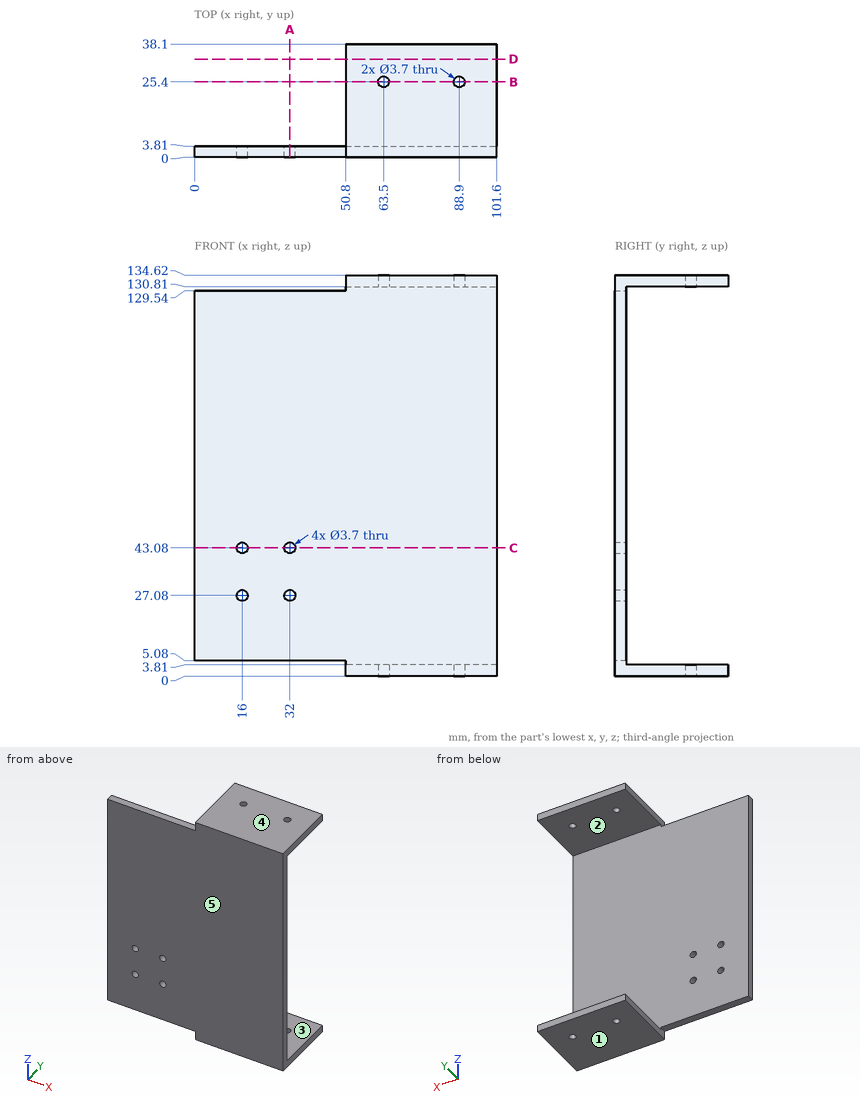
Part print with two shaded views. Sizes in mm from the minimum x, y, z corner. A direction names the side the tool comes from. Coordinates: 2 decimals unless noted, no trailing zeros. Order: outer loops, then holes, each group sorted by start corner. A loop starts at its lowest first (then second) coordinate and runs counter-clockwise, first axis right, second up. Notation, with made-up numbers: M 61.25,51 L 105.25,51 A33 ccw 105.25,87 Z; hole C -24.75,62.25 d9. An arc over 180 degrees is marked long. One line per question, with ' | ' between items. Start each with the question number.
1. Cut at D-D (y = 33). Write the cut outline in (x, z), plus the area to 3 significant figures.
2. Cut at B-B (y = 25.4). Write the cut outline in (x, z).
3. Mould opens along Z. For the marked faces 3, 4 and 5 say: +Z half, -Z half, draft (parallel to the pull), parting line (faces both ways), or undercut.
4. Tool access for the marked faces 1 and 2: list every direction of +Z, -Z, +X, -X, +Y, -Y with a clear straight run to the whole face (end or side of a thin tool).
5. Cut at A-A (x = 32). Write the cut outline in (y, z), plus the area to 3 significant figures.
6. Cut at C-C (z = 43.08). Write the cut outline in (x, y).
7. Flat gauge pins, fed straight in: P1, Ø2, axis at x = 88.9, y = 25.4, coming from the -Z side; P2, Ø2.5, axis at y = 27.5, z = 132, coming from the -X side; P3, Ø5, axis at x = 32, z = 27.08, coming from the +Y side; P4, Ø1.9, axis at x = 28.5, y = 1.5, coming from the -Z side. Where does each tip first touch, or does it go through?
8. Wall check: line 1 along X through (y, z) = (1.35, 43.08); line 2 along X through (y, z) = (25.4, 2.25); line 3 along Z through (x, y) = (16, 2.2). Give the ranges that are in metal, low to high. Write a range as [from, to].
The answers:
1) outline: M 50.8,0 L 101.6,0 L 101.6,3.81 L 50.8,3.81 Z; M 50.8,130.81 L 101.6,130.81 L 101.6,134.62 L 50.8,134.62 Z | area: 387 mm2
2) outline: M 50.8,0 L 61.65,0 L 61.65,3.81 L 50.8,3.81 Z; M 50.8,130.81 L 61.65,130.81 L 61.65,134.62 L 50.8,134.62 Z; M 65.35,0 L 87.05,0 L 87.05,3.81 L 65.35,3.81 Z; M 65.35,130.81 L 87.05,130.81 L 87.05,134.62 L 65.35,134.62 Z; M 90.75,0 L 101.6,0 L 101.6,3.81 L 90.75,3.81 Z; M 90.75,130.81 L 101.6,130.81 L 101.6,134.62 L 90.75,134.62 Z
3) face 3: undercut | face 4: +Z half | face 5: draft
4) face 1: -Z, +X, -X, +Y, -Y | face 2: +X, -X, +Y
5) outline: M 0,5.08 L 3.81,5.08 L 3.81,25.23 L 0,25.23 Z; M 0,28.93 L 3.81,28.93 L 3.81,41.23 L 0,41.23 Z; M 0,44.93 L 3.81,44.93 L 3.81,129.54 L 0,129.54 Z | area: 446 mm2
6) outline: M 0,0 L 14.15,0 L 14.15,3.81 L 0,3.81 Z; M 17.85,0 L 30.15,0 L 30.15,3.81 L 17.85,3.81 Z; M 33.85,0 L 101.6,0 L 101.6,3.81 L 33.85,3.81 Z
7) P1: passes through | P2: stops at x = 50.8 | P3: stops at y = 3.81 | P4: stops at z = 5.08
8) line 1: x = [0, 14.15], [17.85, 30.15], [33.85, 101.6] | line 2: x = [50.8, 61.65], [65.35, 87.05], [90.75, 101.6] | line 3: z = [5.08, 25.23], [28.93, 41.23], [44.93, 129.54]
